from build123d import *

# Parameters (mm, degrees)
F2_R    = 5
F3_SIZE = 0.5


with BuildPart() as f1:
    # F0 (on Front) → F1 (revolve)
    with BuildSketch(Plane.XZ):
        Polygon((-43, 35), (-43, 32.5), (43, 32.5), (43, 35), (40, 38), (40, 70), (-40, 70), (-40, 38), align=None)
    revolve(axis=Axis((10.727409, 0, 0), (1, 0, 0)))

    # F2
    f2_edges = [f1.edges().sort_by_distance(p)[0] for p in [
        (-40, 0, -70),
        (40, 0, -70),
    ]]
    fillet(f2_edges, radius=F2_R)

    # F3
    f3_edges = [f1.edges().sort_by_distance(p)[0] for p in [
        (-43, 0, -32.5),
        (43, 0, -32.5),
        (0, 0, 32.5),
    ]]
    chamfer(f3_edges, length=F3_SIZE)


solid = f1.part
Geometry check sheet. Reference: the model listing, model coordinates, mm. A direction names the side the tool comes from. Coordinates: 2 decimals unless noted, no trailing zeros. Loops run counter-clockwise (first coordinate to the right, second up) from the corner with the lowest first, then second, coordinate; pieces in that order, holes last. Notation, with made-up numbers: (-2.75, 3) - (25.25, 3) arc R18 cw to (25.25, 18) - close; hole circle Ø3 at (-34, 15). An arc over 180 degrees is marked (long way). Use one line per item in the form item = value. Start each with the question number.
Item 1: Section check C-C, the plane x = 4. Enter the section's corners in (y, z).
Item 2: Thickness scan on probe 1 along Z at (x, y) = (15, 0); probe 2 along X at (y, z) = (23.5, -31). Record the ranges inside material, lowest first.
Item 3: Section check A-A, the plane z = 0. Enter the section's corners in (x, y), and give its area (3 significant figures).
Item 4: Gauge pin test, flat ends, axial feed: pin 1 (2 mm diameter, centred on x = 12.5, z = -8, fed in from +Y); pin 2 (6 mm diameter, centred on y = 32.5, z = -54.5, fed in from +X); pin 3 (1 mm diameter, centred on x = -4.5, y = 28.5, fed in from -Z); pin 4 (8 mm diameter, centred on y = -23.5, z = 10, fed in from +X). Record the tip position at first contact, or that the pin passes through.
Item 5: Mould release check, pull along Z, two halves, no side actions. Record for faces 3 (the face through (0.59, -9.76, 31)), 4 (the face through (-42.854, 34.31, -7.619)), 5 (the face through (-40, 28, 28)): +Z half, -Z half, draft (parallel to the pull), parting line (faces both ways), or undercut.
Item 6: Tool access check on faces 1 (the face through (-0.49, 42.594, -55.55)), 2 (the face through (40, 28, -28)). Record the directions out of +Z, -Z, +X, -X, +Y, -Y that give a thin tool (end or side, any length) a straight path to the whole face; none if there is none.
Computed:
q1.outline = circle Ø140 at (0, 0); hole circle Ø65 at (0, 0)
q2.probe_1 = -70 to -32.5, 32.5 to 70
q2.probe_2 = -40 to 40
q3.outline = (-43, -35) - (-40, -38) - (-40, -65) arc R5 ccw to (-35, -70) - (35, -70) arc R5 ccw to (40, -65) - (40, -38) - (43, -35) - (43, -33) - (42.5, -32.5) - (-42.5, -32.5) - (-43, -33) - close; (-43, 33) - (-42.5, 32.5) - (42.5, 32.5) - (43, 33) - (43, 35) - (40, 38) - (40, 65) arc R5 ccw to (35, 70) - (-35, 70) arc R5 ccw to (-40, 65) - (-40, 38) - (-43, 35) - close
q3.area = 6,030 mm2
q4.pin_1 = 69.65
q4.pin_2 = 40
q4.pin_3 = -64.16
q4.pin_4 = through
q5.face_3 = undercut
q5.face_4 = parting line
q5.face_5 = draft
q6.face_1 = +X, -X
q6.face_2 = +X
